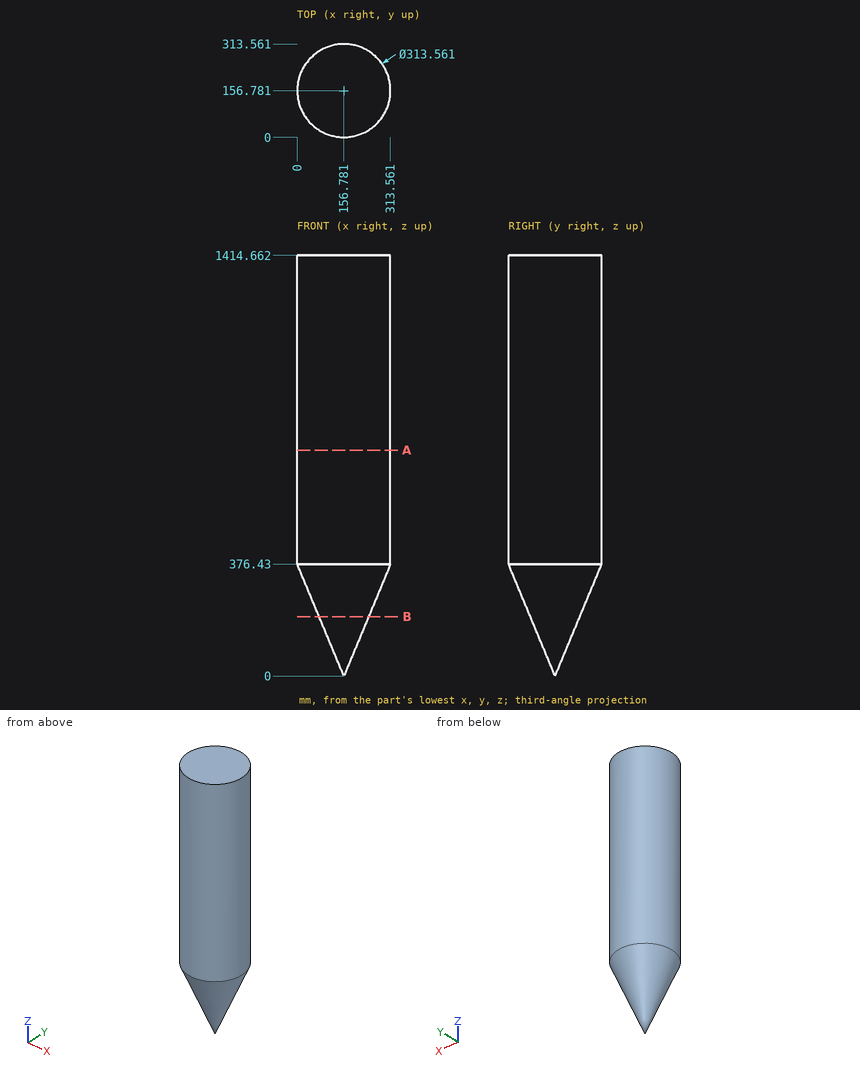
Verification items for this drawing (mm, ordinates from the low corner). Give positions to 0.01 mm unless a question says otherwise; leave off trailing zeros. Write each loop counter-clockwise with the first axis right and the second up, starting at its lowest first coordinate (ties: lowest second). Pieces come first, ordered by that corner, then holes. Notation, with made-up numbers: (72, 4) -> (83, 4) arc R15 ccw to (83, 10) -> close; hole circle Ø9 at (77, -21). An arc over 180 degrees is marked (long way). Use CSV: the item, a comma, the result in double quotes.
(1) Go/stop test with flat-tipped pins: pin 1 (12 mm diameter, centred on x = 141.5, z = 1088, fed in from -Y) (1 decimal); pin 2 (5 mm diameter, centred on x = 31.5, y = 164.5, fed in from -Z) (1 decimal); pin 3 (2 mm diameter, centred on y = 129, z = 696.5, fed in from +X). Record where each tip stops, or that it passes through.
Derived:
pin 1,"stops at y = 0.3"
pin 2,"stops at z = 295.4"
pin 3,"stops at x = 311.26"
(2) Material ranges on L1, parallel to Y at x = 176.5, z = 1220 (1 decimal); L2, parallel to Y at x = 277, z = 889.5 (1 decimal); L3, parallel to Z at x = 245, y = 247.5 (1 decimal), recorded low to high.
Derived:
L1,"y = 1.2 to 312.3"
L2,"y = 56.1 to 257.4"
L3,"z = 303.8 to 1414.7"
(3) Sectioned sample at A-A (z = 759.5). Record the cut outline in (x, y), plus the area to 3 significant figures.
Derived:
outline,"circle Ø313.56 at (156.78, 156.78)"
area,"77,200 mm^2"
(4) Sectioned sample at B-B (z = 199.5). Record the cut outline in (x, y).
Derived:
outline,"circle Ø166.18 at (156.78, 156.78)"
